Here's the drawing with two shaded views (mm, measured from the low corner). I have some questions. Round coordinates to 2 decimals unless told otherwise and drop trailing zeros. Order: outer loops, then holes, each group sorted by start corner. A loop starts at its lowest first (then second) coordinate and runs counter-clockwise, first axis right, second up. Notation, with made-up numbers: (6.5, 86.5) - (15.5, 86.5) arc R10 ccw to (15.5, 98.5) - close; hole circle Ø2 at (35.25, 54). An arc over 180 degrees is marked (long way). Return JSON: item names as keys, results as strings. Group by question number.
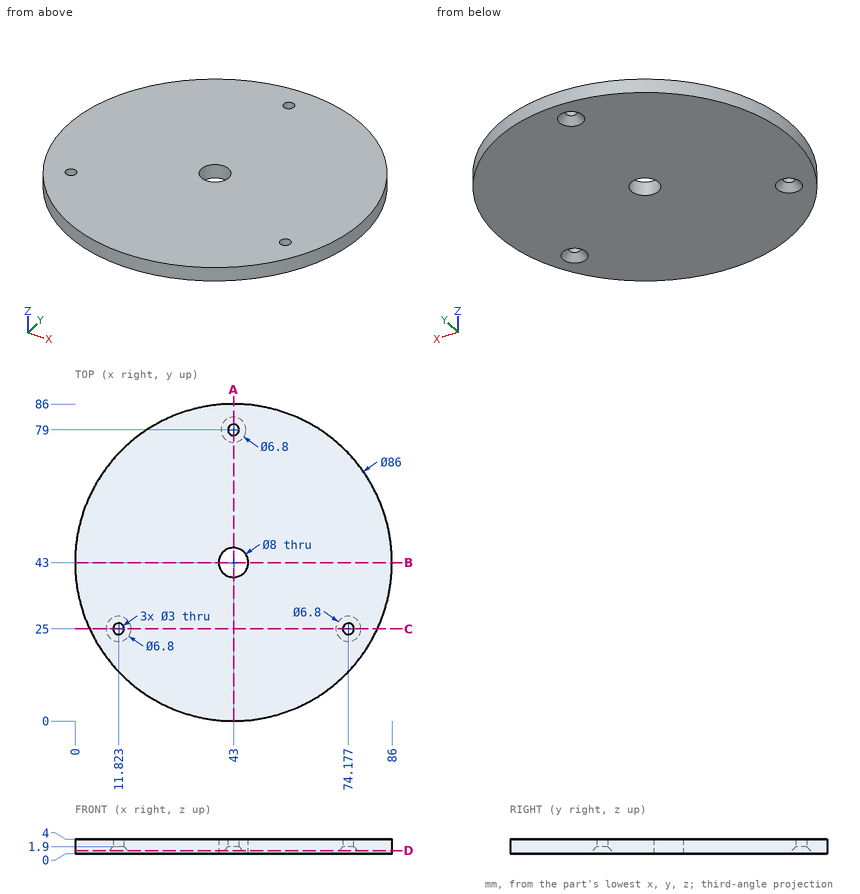
1) Will these pins go through, and if not, where does the flat tip stop? pin 1 (1.5 mm diameter, centred on y = 74.5, z = 0.5, fed in from -X); pin 2 (1.5 mm diameter, centred on y = 26, z = 2, fed in from +X); pin 3 (1.5 mm diameter, centred on x = 59, z = 2, fed in from +Y) (3 decimals).
2) If I drill on line 1 along Y through (x, z) = (43, 3.3); line 2 along Y through (x, z) = (43.5, 1.15); line 3 along X through (y, z) = (6, 2.65), over which ranges is the centre line in solid material (lowest first)? Write a range as from..to.
3) I want a section at C-C, the plane y = 25. List the corners of the cut face in (x, z) for me, plus the area to 3 significant figures.
4) I want a section at A-A, the plane x = 43. List the corners of the cut face in (y, z) for me, plus the area to 3 significant figures.
5) I want a section at B-B, the plane y = 43. List the corners of the cut face in (x, z) for me, plus the area to 3 significant figures.
6) I want a section at D-D, the plane z = 0.85. List the corners of the cut face in (x, y) for me.
Outcome:
{
 "1": {"pin 1": "x = 12.94", "pin 2": "x = 82.81", "pin 3": "y = 83.205"},
 "2": {"line 1": "0..39, 47..77.5, 80.5..86", "line 2": "0..39.03, 46.97..76.81, 81.19..86", "line 3": "21.09..64.91"},
 "3": {"outline": "(3.95, 0) - (8.42, 0) - (10.32, 1.9) - (10.32, 4) - (3.95, 4) - close; (13.32, 1.9) - (15.22, 0) - (70.78, 0) - (72.68, 1.9) - (72.68, 4) - (13.32, 4) - close; (75.68, 1.9) - (77.58, 0) - (82.05, 0) - (82.05, 4) - (75.68, 4) - close", "area": "281 mm^2"},
 "4": {"outline": "(0, 0) - (39, 0) - (39, 4) - (0, 4) - close; (47, 0) - (75.6, 0) - (77.5, 1.9) - (77.5, 4) - (47, 4) - close; (80.5, 1.9) - (82.4, 0) - (86, 0) - (86, 4) - (80.5, 4) - close", "area": "296 mm^2"},
 "5": {"outline": "(0, 0) - (39, 0) - (39, 4) - (0, 4) - close; (47, 0) - (86, 0) - (86, 4) - (47, 4) - close", "area": "312 mm^2"},
 "6": {"outline": "circle Ø86 at (43, 43); hole circle Ø5.1 at (11.82, 25); hole circle Ø8 at (43, 43); hole circle Ø5.1 at (43, 79); hole circle Ø5.1 at (74.18, 25)"}
}
